Geometry: see drawing. Coordinates: mm, zero at the bounding-box minimum. Coordinates: 2 decimals unless noted, no trailing zeros. Write each loop counter-clockwise with the first axis right and the second up, starting at its lowest first coordinate (ties: lowest second). Pieces come first, ordered by that corner, then holes. Notation, with made-up numbers: M -15,3 L 42,3 A37 ccw 42,40 Z; hole C -25.75,-37 d8. An arc over 180 degrees is marked long. One line per item, written item: value. Start each with the question number.
Item 1: Ray query, L1, parallel to Y at x = 4, z = 9; L2, parallel to Y at x = 4.5, z = 12; L3, parallel to X at y = 5, z = 21. Return the intervals inside material, ascending. Write a range as from..to.
Item 2: Cut plane A-A, the plane y = 4. Output: boundary loops of the cut face in (x, z), then the cut area to 3 significant figures.
Item 3: Pin query (flat end, axial travel): P1, Ø1.5, axis at y = 5, z = 12.5, coming from the -X side; P2, Ø3, axis at x = 4, y = 4, coming from the -Z side. Return the tip coordinate at first contact, or that it passes through.
Item 4: Cut plane C-C, the plane z = 5.75. Output: boundary loops of the cut face in (x, y).
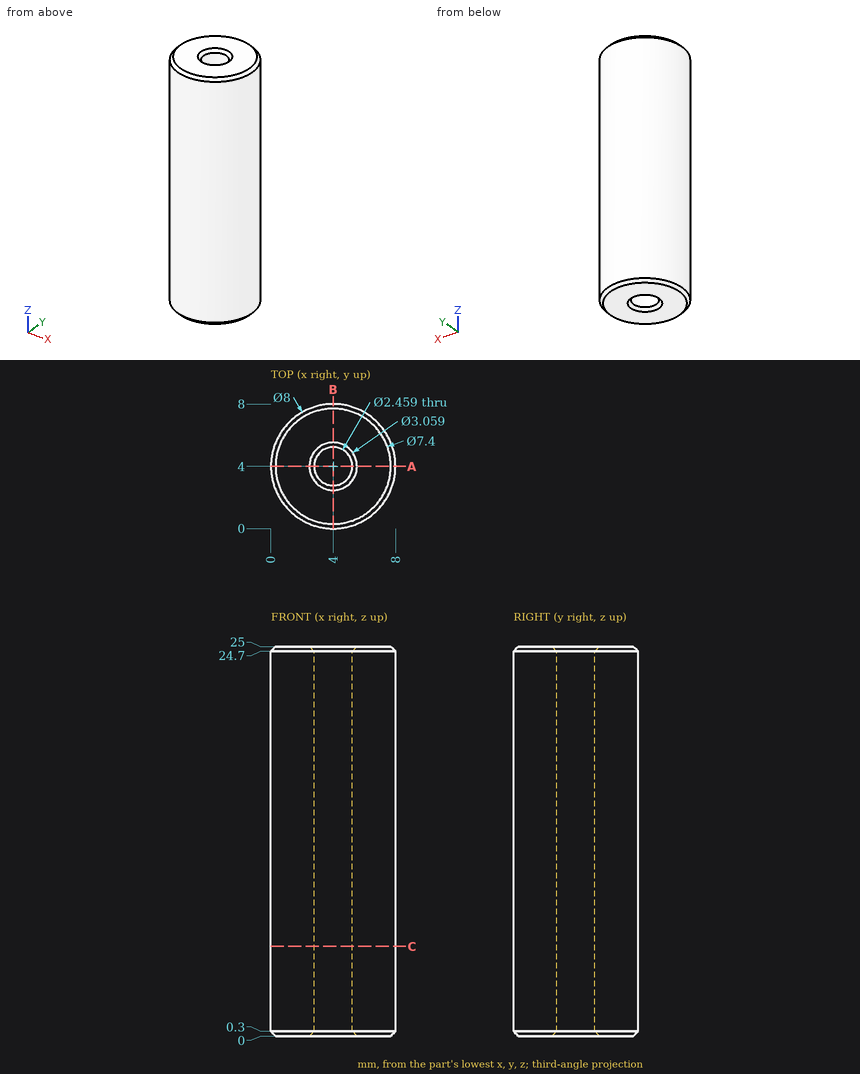
From the geometry:
1. L1: y = 0..2.77, 5.23..8
1. L2: y = 0.03..2.88, 5.12..7.97
1. L3: x = 0.13..3.28, 4.72..7.87
2. outline: M 0,0.3 L 0.3,0 L 2.47,0 L 2.77,0.3 L 2.77,24.7 L 2.47,25 L 0.3,25 L 0,24.7 Z; M 5.23,0.3 L 5.53,0 L 7.7,0 L 8,0.3 L 8,24.7 L 7.7,25 L 5.53,25 L 5.23,24.7 Z
2. area: 138 mm²
3. P1: stops at x = 0.01
3. P2: stops at z = 0.03
4. outline: C 4,4 d8; hole C 4,4 d2.46
